from build123d import *

# Parameters (mm, degrees)
SKETCH001_R      = 1.125
EXTRUDE001_DEPTH = 10
SKETCH_R         = 1.125
EXTRUDE_DEPTH    = 10
TUBE001_R        = 40
TUBE001_R_2      = 30
TUBE001_DEPTH    = 10
TUBE_R           = 50
TUBE_R_2         = 40
TUBE_DEPTH       = 70


with BuildPart() as extrude001:
    # Sketch001 (on Face21 of Fusion001) → Extrude001 (new body)
    with BuildSketch(Plane.XY.offset(70)):
        with Locations((0, 35)):
            Circle(SKETCH001_R)
        with Locations((0, -35)):
            Circle(SKETCH001_R)
    extrude(amount=-EXTRUDE001_DEPTH)


with BuildPart() as extrude_body:
    # Sketch (on Face3 of Tube) → Extrude (new body)
    with BuildSketch(Plane(origin=(0, 0, 0), x_dir=(1, 0, 0), z_dir=(0, 0, -1))):
        Polygon((7.5, 49.4343), (7.5, 64.4343), (0, 64.4343), (-7.5, 64.4343), (-7.5, 49.4343), (0, 49.4343), align=None)
        with Locations((0, 56.9343)):
            Circle(SKETCH_R, mode=Mode.SUBTRACT)
        Polygon((7.5, -49.4343), (7.5, -64.4343), (0, -64.4343), (-7.5, -64.4343), (-7.5, -49.4343), (0, -49.4343), align=None)
        with Locations((0, -56.9343)):
            Circle(SKETCH_R, mode=Mode.SUBTRACT)
    extrude(amount=-EXTRUDE_DEPTH)


with BuildPart() as tube001:
    # Tube001 → Tube001 (new body)
    with BuildSketch(Plane.XY.offset(60)):
        Circle(TUBE001_R)
        Circle(TUBE001_R_2, mode=Mode.SUBTRACT)
    extrude(amount=TUBE001_DEPTH)


with BuildPart() as bigredbuttonmount001:
    # Tube → Tube (new body)
    with BuildSketch(Plane.XY):
        Circle(TUBE_R)
        Circle(TUBE_R_2, mode=Mode.SUBTRACT)
    extrude(amount=TUBE_DEPTH)

    # Fusion: union Tube001
    add(tube001.part)

    # Fusion001: union Extrude body
    add(extrude_body.part)

    # Cut: cut Extrude001
    add(extrude001.part, mode=Mode.SUBTRACT)


solid = bigredbuttonmount001.part
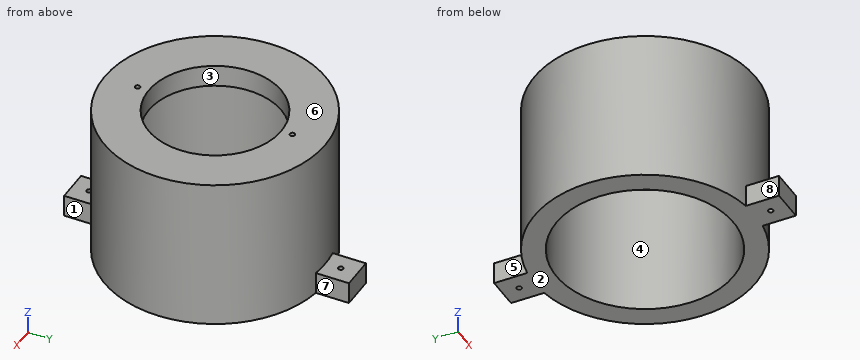
Could you check a few things on this model? Use its own coordinates, in mm. Face numbers are marked on the shaded views. A direction names the side the tool comes from. Coordinates: 2 decimals unless noted, no trailing zeros. Order: outer loops, then holes, each group sorted by start corner. A loop starts at its lowest first (then second) coordinate and runs counter-clockwise, first axis right, second up. Notation, with made-up numbers: (-9.75, -14.5) -> (28.25, -14.5) arc R21 ccw to (28.25, 2.5) -> close; hole circle Ø4 at (15.5, 26). An arc over 180 degrees is marked (long way). One line per question, with ' | ' between items.
Q1. Thinking about a two-plate mould opening in X: for the marked faces 1, 2 and 3, which applies, pulls with the +X half, pulls with the -X half, needs draft (parallel to the pull), parting line crosses it, or undercut?
Return value:
face 1: pulls with the +X half | face 2: needs draft | face 3: undercut
Q2. Imagine slicing it at B-B on x = 17.5. Please give me the cut outline in (y, z), and give its area (3 significant figures).
Return value:
outline: (-46.84, 0) -> (-35.97, 0) -> (-35.97, 60) -> (-24.37, 60) -> (-24.37, 70) -> (-46.84, 70) -> close; (24.37, 60) -> (35.97, 60) -> (35.97, 0) -> (46.84, 0) -> (46.84, 70) -> (24.37, 70) -> close | area: 1,750 mm²
Q3. I'm going to push flat-ended pins straight in: P1, Ø10, axis at y = 31.5, z = 9, coming from the +X side; P2, Ø4, axis at x = 36, z = 33.5, coming from the +Y side; P3, Ø11, axis at y = 59, z = 6.5, coming from the -X side; P4, Ø24, axis at x = 17, y = 0, coming from the -Z side. Where does each tip first touch, or does it pass through?
Return value:
P1: x = 42.4 | P2: y = 36.66 | P3: x = -7.5 | P4: through
Q4. On a 3-axis mill with a long thin cutter (end or side, diameter ignored), from which of +Z, -Z, +X, -X, +Y, -Y can I reach the whole of each face in a straight line? I mean the marked faces 4, 5, 6, 7 and 8. Say none if no direction works.
Return value:
face 4: -Z | face 5: +Z, -Z, -X, +Y | face 6: +Z, +X, -X, +Y, -Y | face 7: +Z, -Z, +X, +Y | face 8: +Z, -Z, -X, -Y
Q5. If I drill on L1, parallel to Y at x = 0, z = 66.5 (3 decimals); L2, parallel to Y at x = 0, z = 4.75; L3, parallel to X at y = 19.5, z = 34, over which ranges is the centre line in solid material (lowest first)?
Return value:
L1: -50 to -36.125, -33.875 to -30, 30 to 33.875, 36.125 to 50 | L2: -64.43 to -58.06, -55.81 to -40, 40 to 55.81, 58.06 to 64.43 | L3: -46.04 to -34.92, 34.92 to 46.04
Q6. Imagine slicing it at C-C on z = 7. Please give me the cut outline in (x, y) (3 decimals).
Return value:
outline: (-7.5, -64.434) -> (7.5, -64.434) -> (7.5, -49.434) arc R50 ccw to (7.5, 49.434) -> (7.5, 64.434) -> (-7.5, 64.434) -> (-7.5, 49.434) arc R50 ccw to (-7.5, -49.434) -> close; hole circle Ø80 at (0, 0); hole circle Ø2.25 at (0, -56.934); hole circle Ø2.25 at (0, 56.934)
Q7. Imagine slicing it at D-D on y = -38. Please give me the cut outline in (x, z).
Return value:
outline: (-32.5, 0) -> (-12.49, 0) -> (-12.49, 60) -> (12.49, 60) -> (12.49, 0) -> (32.5, 0) -> (32.5, 70) -> (-32.5, 70) -> close
Q8. Imagine slicing it at A-A on y = 0. Please give me the cut outline in (x, z), and give its area (3 significant figures).
Return value:
outline: (-50, 0) -> (-40, 0) -> (-40, 60) -> (-30, 60) -> (-30, 70) -> (-50, 70) -> close; (30, 60) -> (40, 60) -> (40, 0) -> (50, 0) -> (50, 70) -> (30, 70) -> close | area: 1,600 mm²
